Geometry: final body of the model. Coordinates: model frame, mm. Face numbers are marked on the shaded views. A direction names the side the tool comes from. Coordinates: 2 decimals unless noted, no trailing zeros. Write each loop counter-clockwise with the first axis right and the second up, starting at its lowest first coordinate (ties: lowest second). Pieces come first, ordered by that corner, then holes. Notation, with made-up numbers: (73.5, 45) - (99.5, 45) arc R18 ccw to (99.5, 73) - close; hole circle Ø11 at (73.25, -2). An arc over 180 degrees is marked (long way). Answer as a JSON object with one key per item and string values. Group by question number.
Item 1: Section A-A on y = 0. Return loops of the section in (x, z), and give its area (3 significant figures).
Item 2: Section B-B on z = 18.5. Return loops of the section in (x, y), and give its area (3 significant figures).
Item 3: Section D-D on x = 100.5. Return loops of the section in (y, z).
Item 4: Set-up query: the marked faces 3 and 4. Return all of +Z, -Z, +X, -X, +Y, -Y with unobstructed straight access to the full face (end or side cutting, diameter ignored); none if empty.
Item 5: Section C-C on z = 53.5. Return loops of the section in (x, y), and give its area (3 significant figures).
Item 6: Line query: line 1 along X through (y, z) = (0, 45.5); line 2 along Y through (x, z) = (52, 61); line 3 along Y through (x, z) = (112, 35). Output: solid intervals per line, ascending. Write a range as from..to.
Item 7: Mould query, pull axis X, two halves, no side actions, for the marked faces 1 and 2. Classes: pulls with the +X half, pulls with the -X half, needs draft (parallel to the pull), parting line crosses it, or undercut.
Item 8: First-contact query: pin 1 Ø3 at (y, z) = (14.5, 71.5) entering from -X; pin 2 Ø1 at (x, y) = (54, -15) entering from +Z; pin 3 Ø5 at (x, z) = (77.5, 7) entering from +Y; pin 4 Ø12 at (y, z) = (3, 48) entering from +X. Flat tips, straight axial feed; report the tip coordinate or a pass-through.
Autodesk Inventor part; units mm, degrees
ref_plane "YZ Plane" through (0, 0, 0) normal (1, 0, 0) x (0, 1, 0)
ref_plane "XZ Plane" through (0, 0, 0) normal (0, 1, 0) x (-1, 0, 0)
ref_plane "XY Plane" through (0, 0, 0) normal (0, 0, 1) x (1, 0, 0)
sketch "Sketch1" plane through (0, 0, 0) normal (1, 0, 0) x (0, 1, 0)
  circle A0 centre (0, 0) radius 44.45
  dimension "d0" = 88.9
extrude "Extrude1" add sketch "Sketch1" along normal blind 172
sketch "Sketch2" plane through (0, 0, 0) normal (0, 0, 1) x (1, 0, 0)
  line L0 (0, 44.45) -> (0, -44.45)
  line L1 (172, 44.45) -> (172, -44.45)
  line L2 (0, 0) -> (172, 0) construction
  circle A0 centre (86, 0) radius 44.45
  dimension "d3" = 88.9
extrude "Extrude2" add sketch "Sketch2" along normal blind 86
sketch "Sketch3" plane through (0, 0, 0) normal (-1, 0, 0) x (0, 0, 1)
  circle A0 centre (0, 0) radius 44.45
  circle A1 centre (0, 0) radius 38.85
  dimension "d6" = 77.7
extrude "Extrude3" cut sketch "Sketch3" against normal through all contours A1
sketch "Sketch4" plane through (86, 0, 86) normal (0, 0, 1) x (1, 0, 0)
  circle A0 centre (0, 0) radius 44.45
  circle A1 centre (0, 0) radius 38.85
  dimension "d9" = 77.7
extrude "Extrude4" cut sketch "Sketch4" against normal up to next contours A1
equation "\"d0\" = d"
equation "\"d1\" = 2 * a"
equation "\"d3\" = d"
equation "\"d4\" = a"
equation "\"d6\" = d - 2 * s1"
equation "\"d7\" = a"
equation "\"d9\" = d - 2 * s1"
equation "\"d10\" = a"
equation "\"d\" = 88.9"
equation "\"s1\" = 5.6"
equation "\"a\" = 86"
equation "\"Size_Designation\" = 1.2345"
properties part number "DIN 2615-1 Tee 88.9 x 5.6 S" material "Steel"
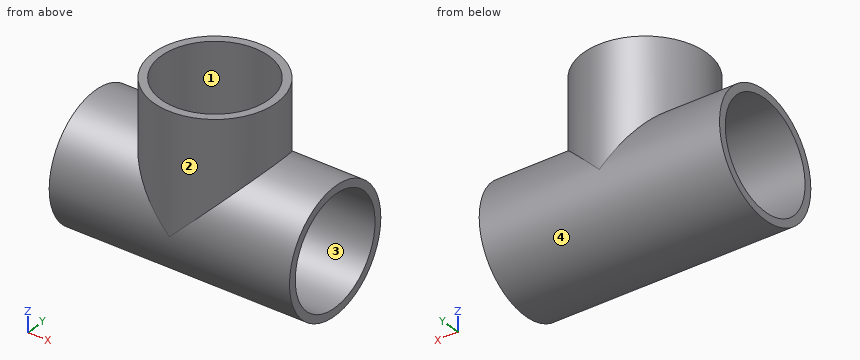
Checks:
{
 "1": {"outline": "(0, -44.45) - (172, -44.45) - (172, -38.85) - (0, -38.85) - close; (0, 38.85) - (47.15, 38.85) - (47.15, 86) - (41.55, 86) - (41.55, 44.45) - (0, 44.45) - close; (124.85, 38.85) - (172, 38.85) - (172, 44.45) - (130.45, 44.45) - (130.45, 86) - (124.85, 86) - close", "area": "1,960 mm^2"},
 "2": {"outline": "(0, -40.42) - (67.5, -40.42) arc R44.45 ccw to (104.5, -40.42) - (172, -40.42) - (172, -34.16) - (104.5, -34.16) arc R38.85 cw to (67.5, -34.16) - (0, -34.16) - close; (0, 34.16) - (67.5, 34.16) arc R38.85 cw to (104.5, 34.16) - (172, 34.16) - (172, 40.42) - (104.5, 40.42) arc R44.45 ccw to (67.5, 40.42) - (0, 40.42) - close", "area": "2,120 mm^2"},
 "3": {"outline": "(-42.02, 14.5) arc R44.45 ccw (long way) to (42.02, 14.5) - (42.02, 86) - (36.04, 86) - (36.04, 14.5) arc R38.85 cw (long way) to (-36.04, 14.5) - (-36.04, 86) - (-42.02, 86) - close"},
 "4": {"face 3": "+X, -X", "face 4": "none"},
 "5": {"outline": "circle Ø88.9 at (86, 0); hole circle Ø77.7 at (86, 0)", "area": "1,470 mm^2"},
 "6": {"line 1": "41.55..47.15, 124.85..130.45", "line 2": "-28.63..-18.8, 18.8..28.63", "line 3": "-36.05..-28.87, 28.87..36.05"},
 "7": {"face 1": "undercut", "face 2": "parting line crosses it"},
 "8": {"pin 1": "x = 43.49", "pin 2": "z = -35.62", "pin 3": "y = 44.22", "pin 4": "x = 172"}
}
